from build123d import *

# Parameters (mm, degrees)
SKETCH_R     = 10.4
PAD_DEPTH    = 43
SKETCH001_R  = 3
PAD001_DEPTH = 2
SKETCH002_R  = 2
PAD002_DEPTH = 11


with BuildPart() as part:
    # Sketch → Pad (new body)
    with BuildSketch(Plane.XY):
        Circle(SKETCH_R)
    extrude(amount=PAD_DEPTH)

    # Sketch001 (on Face3 of Pad) → Pad001 (join)
    with BuildSketch(Plane.XY.offset(43)):
        Circle(SKETCH001_R)
    extrude(amount=PAD001_DEPTH)

    # Sketch002 (on Face5 of Pad001) → Pad002 (join)
    with BuildSketch(Plane.XY.offset(45)):
        Circle(SKETCH002_R)
    extrude(amount=PAD002_DEPTH)


with BuildPart() as part_1:
    # Body placement: moved
    add(part.part.moved(Location((0, -8, 0))))


solid = part_1.part
Could you check a few things on this model? Use its own coordinates, in mm. A direction names the side the tool comes from. Coordinates: 2 decimals unless noted, no trailing zeros. Order: outer loops, then holes, each group sorted by start corner. A loop starts at its lowest first (then second) coordinate and runs counter-clockwise, first axis right, second up. Notation, with made-up numbers: (18, 76) - (46, 76) arc R7 ccw to (46, 81) - close; hole circle Ø8 at (-33, 42). An arc over 180 degrees is marked (long way). Answer in a Markdown table with one row per item. Add a question column.
(1) I need wall thicknesses on L1, parallel to Y at x = -0.5, z = 41.5; L2, parallel to Z at x = -2.5, y = -9.5; L3, parallel to Z at x = 4.5, y = -15. Which ranges of each line are inside material? Lowest first, please.
(2) If we section it at A-A, the plane y = -8: Please give me the cut outline in (x, z).
(3) If we section it at D-D, the plane z = 46.5: Please give me the cut outline in (x, y), then the cut area to 3 significant figures.
(4) Will these pins go through, and if not, where does the flat tip stop? pin 1 (1 mm diameter, centred on y = -10.5, z = 27.5, fed in from -X); pin 2 (10 mm diameter, centred on x = 7, z = 42.5, fed in from +Y); pin 3 (4 mm diameter, centred on y = -13, z = 46, fed in from -X); pin 4 (5 mm diameter, centred on y = -15.5, z = 28, fed in from +X).
(5) On a 3-axis mill with a long thin cutter (end or side, diameter ignored), from which of +Z, -Z, +X, -X, +Y, -Y can I reach the whole of each face in a straight line? I mean faces 1 (the face through (0, -5, 44)), 2 (the face through (4.799, -17.227, 21.199)). Say none if no direction works.
(6) If we section it at B-B, the plane x = 0: Please give me the cut outline in (y, z).
(7) If we section it at C-C, the plane z = 34.5: Please give me the cut outline in (x, y), then the cut area to 3 significant figures.
Results are:
| question | item | result |
|---|---|---|
| 1 | L1 | y = -18.39 to 2.39 |
| 1 | L2 | z = 0 to 45 |
| 1 | L3 | z = 0 to 43 |
| 2 | outline | (-10.4, 0) - (10.4, 0) - (10.4, 43) - (3, 43) - (3, 45) - (2, 45) - (2, 56) - (-2, 56) - (-2, 45) - (-3, 45) - (-3, 43) - (-10.4, 43) - close |
| 3 | outline | circle Ø4 at (0, -8) |
| 3 | area | 12.6 mm2 |
| 4 | pin 1 | stops at x = -10.21 |
| 4 | pin 2 | stops at y = 2.21 |
| 4 | pin 3 | passes through |
| 4 | pin 4 | stops at x = 9.12 |
| 5 | face 1 | +Z |
| 5 | face 2 | +Z, -Z |
| 6 | outline | (-18.4, 0) - (2.4, 0) - (2.4, 43) - (-5, 43) - (-5, 45) - (-6, 45) - (-6, 56) - (-10, 56) - (-10, 45) - (-11, 45) - (-11, 43) - (-18.4, 43) - close |
| 7 | outline | circle Ø20.8 at (0, -8) |
| 7 | area | 340 mm2 |
